Answer from the drawing. Dimensions are ordinates in mm from the lowest x, y and z of the part. Round coordinates to 2 decimals unless told otherwise and drop trailing zeros. Write each loop counter-clockwise with the first axis right and the second up, starting at its lowest first coordinate (ties: lowest second). Pieces come first, ordered by that corner, then holes. Notation, with made-up numbers: (1.25, -38) - (23.25, -38) arc R31 ccw to (23.25, -10) - close; hole circle Ø11 at (30, 47). An arc over 180 degrees is marked (long way). Return JSON: item names as keys, results as strings. Group by question number.
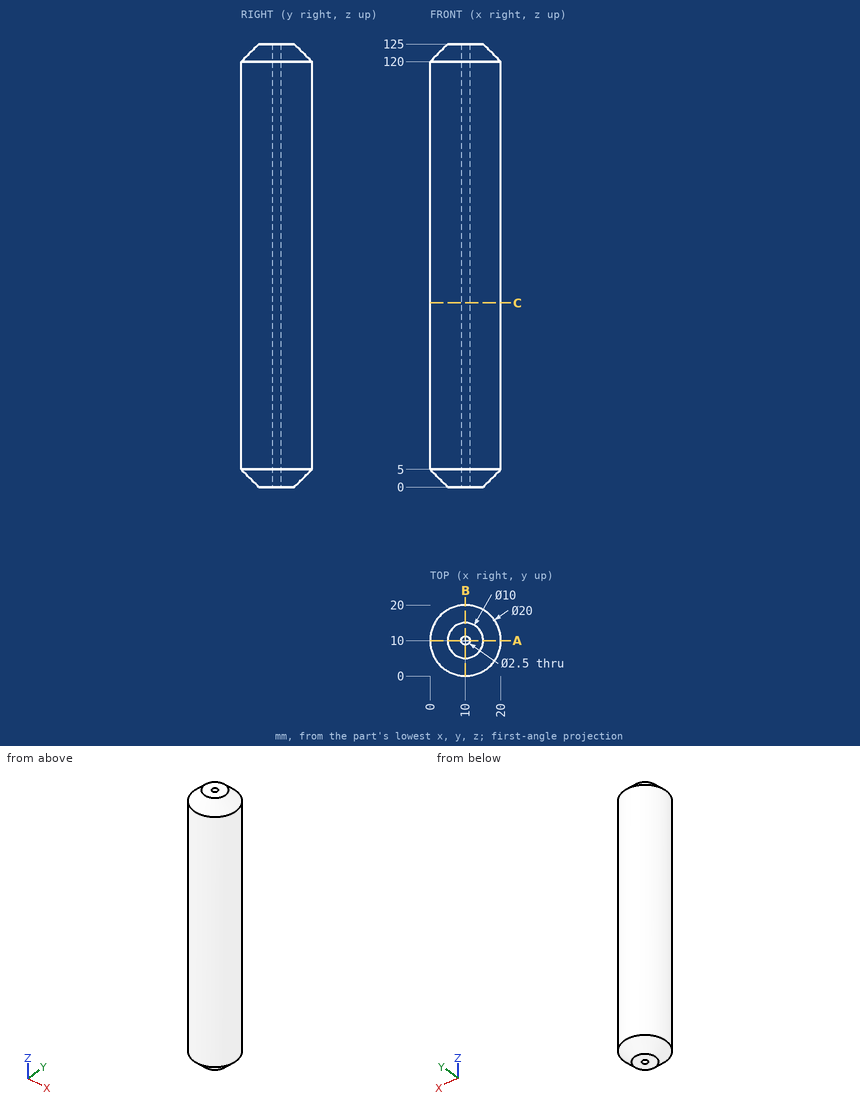
(1) Flat-ended cylindrical pins translate along their axes: pin 1 (1.5 mm diameter, centred on y = 12, z = 101.5, fed in from +X); pin 2 (4 mm diameter, centred on x = 4, y = 3, fed in from -Z); pin 3 (4 mm diameter, centred on x = 13, z = 52.5, fed in from -Y). Find the tip coordinate at first contact, or state that the pin passes through.
(2) Find section C-C (z = 52). Write down the section's boundary in (x, y), plus the area to 3 significant figures.
(3) Find section A-A (y = 10). Write down the section's boundary in (x, z), plus the area to 3 significant figures.
(4) Consider line 1 (Y direction, x = 10, z = 39.5); line 2 (Y direction, x = 12.5, z = 56.5); line 3 (X direction, y = 18, z = 27). Determine where each line is inside the solid, lowest interval first.
Check sheet entries:
{
 "1": {"pin 1": "stops at x = 19.92", "pin 2": "stops at z = 2.22", "pin 3": "stops at y = 0.05"},
 "2": {"outline": "circle Ø20 at (10, 10); hole circle Ø2.5 at (10, 10)", "area": "309 mm^2"},
 "3": {"outline": "(0, 5) - (5, 0) - (8.75, 0) - (8.75, 125) - (5, 125) - (0, 120) - close; (11.25, 0) - (15, 0) - (20, 5) - (20, 120) - (15, 125) - (11.25, 125) - close", "area": "2,140 mm^2"},
 "4": {"line 1": "y = 0 to 8.75, 11.25 to 20", "line 2": "y = 0.32 to 19.68", "line 3": "x = 4 to 16"}
}
